Geometry: final body of the model. Coordinates: model frame, mm. Face numbers are marked on the shaded views. A direction names the side the tool comes from. Give positions to 0.01 mm unless a question says otherwise; leave off trailing zeros. Order: outer loops, then holes, each group sorted by start corner. A loop starts at its lowest first (then second) coordinate and runs counter-clockwise, first axis right, second up. Notation, with made-up numbers: (80, -11.75) - (128, -11.75) arc R28 cw to (128, 18.25) - close; hole circle Ø6 at (47.25, 35.25). An arc over 180 degrees is marked (long way). Write item = value, one per line. Start each with the question number.
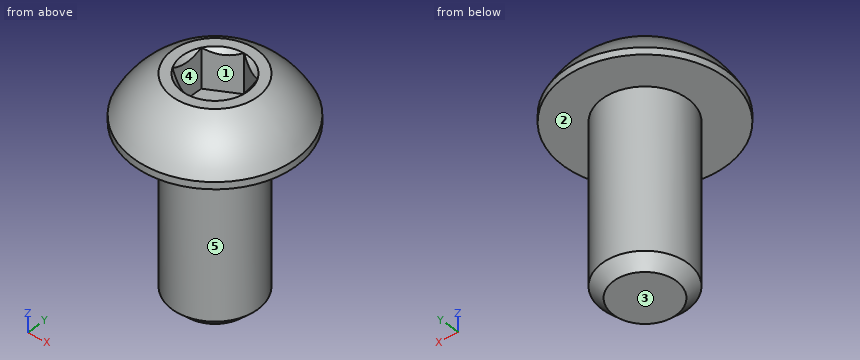
from build123d import *

# Parameters (mm, degrees)
CUT_EXTRUDE1_DEPTH = 1.4


with BuildPart() as part:
    # Sketch2 → Revolve1 (revolve)
    with BuildSketch(Plane(origin=(0, 0, 0), x_dir=(0, 0, -1), z_dir=(1, 0, 0)), mode=Mode.PRIVATE) as revolve1_sk:
        with BuildLine():
            Line((-3.825, 0), (3.825, 0))
            Line((3.825, 0), (3.825, 1.1))
            Line((3.825, 1.1), (3.425, 1.5))
            Line((3.425, 1.5), (-2.175, 1.5))
            Line((-2.175, 1.5), (-2.175, 2.85))
            Line((-2.175, 2.85), (-2.4225, 2.85))
            ThreePointArc((-2.4225, 2.85), (-3.22987489, 2.285251969), (-3.825, 1.5))
            Line((-3.825, 1.5), (-3.825, 0))
        make_face()
    revolve(revolve1_sk.sketch.rotate(Axis((0, 0, 3.825), (0, 0, -1)), 90), axis=Axis((0, 0, 3.825), (0, 0, -1)))

    # Sketch3 → Cut-Extrude1 (cut)
    with BuildSketch(Plane.XY.offset(3.825)):
        Polygon((0, 1.154700538), (-1, 0.577350269), (-1, -0.577350269), (0, -1.154700538), (1, -0.577350269), (1, 0.577350269), align=None)
    extrude(amount=-CUT_EXTRUDE1_DEPTH, mode=Mode.SUBTRACT)

    # Cut-Extrude2 cone 1 section (through the dimple's axis) → Cut-Extrude2 (revolve, cut)
    with BuildSketch(Plane(origin=(0, 0, 3.825), x_dir=(0, -1, 0), z_dir=(1, 0, 0))):
        Polygon((0, 0), (1.154700538, 0), (0, 1.154700538), align=None)
    revolve(axis=Axis((0, 0, 3.825), (0, 0, -1)), mode=Mode.SUBTRACT)


solid = part.part
Q1. Section B-B, the plane z = 1.5. Return the cut outline in (x, y), then the cut area to 3 significant figures.
Q2. Contact query for flat-ended pins moving along their axis: pin 1 (1 mm diameter, centred on x = 1.5, z = 1.5, fed in from +Y); pin 2 (0.9 mm diameter, centred on y = 0, z = 3, fed in from +X); pin 3 (0.6 mm diameter, centred on y = 0, z = 3.5, fed in from -X). Output: stop coordinate, or through.
Q3. Set-up query: the marked faces 1 and 2. Return all of +Z, -Z, +X, -X, +Y, -Y with unobstructed straight access to the full face (end or side cutting, diameter ignored); none if empty.
Q4. Material intervals for line 1 along X through (y, z) = (0.2, 3.75); line 2 along Z through (x, y) = (-0.1, -0.6) (3 decimals); line 3 along X through (y, z) = (0.3, 1.75), sorted ascending. Write a range as from..to.
Q5. Pull-direction query (X, two-part tool) for the marked faces 3, 4 and 5; classes: +X half, -X half, draft (parallel to the pull), parting line (faces both ways), or undercut.
The answers:
q1.outline = circle Ø3 at (0, 0)
q1.area = 7.07 mm²
q2.pin_1 = 1.12
q2.pin_2 = 2.78
q2.pin_3 = -2.31
q3.face_1 = +Z
q3.face_2 = -Z
q4.line_1 = -1.62..-1.06, 1.06..1.62
q4.line_2 = -3.825..2.425
q4.line_3 = -1.47..1.47
q5.face_3 = draft
q5.face_4 = undercut
q5.face_5 = parting line
